Check sheet for the drawn part. Datum: minimum x, y, z corner. Units: mm. A direction names the side the tool comes from. Round coordinates to 2 decimals unless told otherwise and drop trailing zeros. Write each loop counter-clockwise with the first axis right and the second up, starting at its lowest first coordinate (ties: lowest second). Pieces come first, ordered by that corner, then holes. Notation, with made-up numbers: (-12.75, 47) -> (-6.75, 47) arc R29 ccw to (-6.75, 86) -> close; hole circle Ø4 at (10, -6.5). An arc over 180 degrees is marked (long way). Use a Markdown table: item, result.
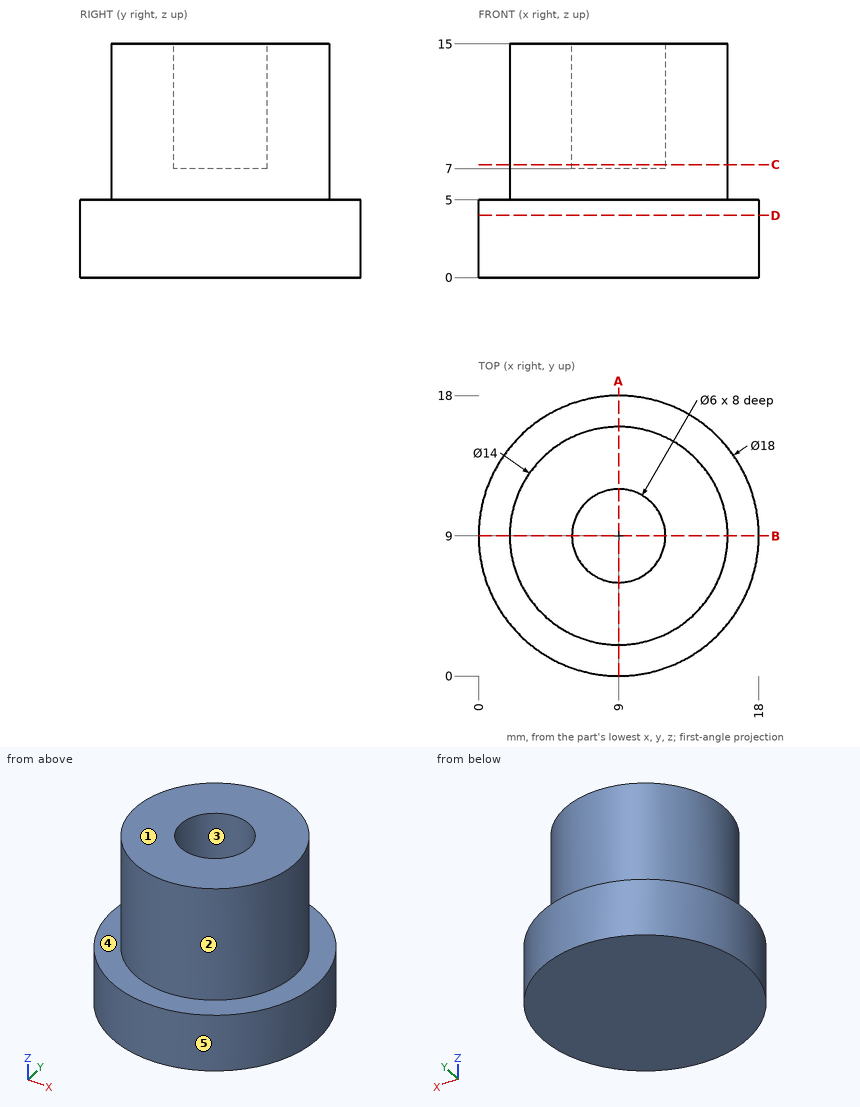
(1) Section check C-C on z = 7.25. Record the cut outline in (x, y), plus the area to 3 significant figures.
A:
| item | result |
|---|---|
| outline | circle Ø14 at (9, 9); hole circle Ø6 at (9, 9) |
| area | 126 mm2 |
(2) Gauge pin test, flat ends, axial feed: pin 1 Ø1.5 at (x, z) = (6.5, 10.5) entering from +Y; pin 2 Ø5 at (x, z) = (12, 8.5) entering from -Y; pin 3 Ø5 at (x, y) = (9, 9) entering from +Z. Record the tip position at first contact, or that the pin passes through.
A:
| item | result |
|---|---|
| pin 1 | stops at y = 15.78 |
| pin 2 | stops at y = 2.02 |
| pin 3 | stops at z = 7 |
(3) Release check for a two-part mould opening along X. For the marked faces 1, 2 and 3 record: +X half, -X half, draft (parallel to the pull), parting line (faces both ways), or undercut.
A:
| item | result |
|---|---|
| face 1 | draft |
| face 2 | parting line |
| face 3 | undercut |
(4) Section check D-D on z = 4. Record the cut outline in (x, y), plus the area to 3 significant figures.
A:
| item | result |
|---|---|
| outline | circle Ø18 at (9, 9) |
| area | 254 mm2 |
(5) Access from +Z, -Z, +X, -X, +Y, -Y to the whole of each face (thin tool, end or side, straight path). Record for the marked faces 4 and 5.
A:
| item | result |
|---|---|
| face 4 | +Z |
| face 5 | +Z, -Z |
(6) Section check A-A on x = 9. Record the cut outline in (y, z).
A:
| item | result |
|---|---|
| outline | (0, 0) -> (18, 0) -> (18, 5) -> (16, 5) -> (16, 15) -> (12, 15) -> (12, 7) -> (6, 7) -> (6, 15) -> (2, 15) -> (2, 5) -> (0, 5) -> close |
(7) Thickness scan on line 1 (Y direction, x = 9, z = 8.5); line 2 (Z direction, x = 1.75, y = 9.75); line 3 (Z direction, x = 9.75, y = 11). Record the ranges inside material, lowest first.
A:
| item | result |
|---|---|
| line 1 | y = 2 to 6, 12 to 16 |
| line 2 | z = 0 to 5 |
| line 3 | z = 0 to 7 |
